Autodesk Inventor part; units mm, degrees
ref_plane "YZ Plane" through (0, 0, 0) normal (1, 0, 0) x (0, 1, 0)
ref_plane "XZ Plane" through (0, 0, 0) normal (0, 1, 0) x (-1, 0, 0)
ref_plane "XY Plane" through (0, 0, 0) normal (0, 0, 1) x (1, 0, 0)
sketch "Sketch1" plane through (0, 0, 0) normal (0, 0, 1) x (1, 0, 0)
  line L0 (0, 0) -> (479.525, 0)
  line L1 (479.525, 0) -> (479.525, 85)
  line L2 (479.525, 85) -> (0, 85)
  line L3 (0, 85) -> (0, 0)
  dimension "d0" = 479.525
  dimension "d1" = 85
extrude "Extrusion1" add sketch "Sketch1" along normal blind 4.7625
sketch "Sketch2" plane through (0, 0, 4.7625) normal (0, 0, 1) x (1, 0, 0)
  line L0 (0, 0) -> (479.525, 0)
  line L1 (382.925, 46.859) -> (382.925, 38.141)
  line L2 (399.525, 38.141) -> (399.525, 46.859)
  arc A0 (382.925, 38.141) -> (399.525, 38.141) centre (391.225, 42.5) ccw
  arc A1 (399.525, 46.859) -> (382.925, 46.859) centre (391.225, 42.5) ccw
  line L3 (479.525, 0) -> (479.525, 85)
  dimension "d5" = 16.6
  dimension "d6" = 9.375
  dimension "d7" = 9.375
  dimension "d8" = 42.5
  dimension "d23" = 80
extrude "Extrusion2" cut sketch "Sketch2" against normal up to next
sketch "Sketch3" plane through (0, 0, 4.7625) normal (0, 0, 1) x (1, 0, 0)
  line L0 (0, 0) -> (479.525, 0)
  line L1 (479.525, 0) -> (479.525, 85)
  line L2 (479.525, 85) -> (0, 85)
  line L3 (0, 85) -> (0, 0)
  circle A0 centre (14.7625, 75) radius 2.25
  circle A1 centre (14.7625, 10) radius 2.25
  circle A2 centre (464.7625, 75) radius 2.25
  circle A3 centre (464.7625, 10) radius 2.25
  circle A4 centre (238.2625, 10) radius 2.25
  circle A5 centre (238.2625, 75) radius 2.25
  dimension "d12" = 4.5
  dimension "d13" = 14.7625
  dimension "d14" = 14.7625
  dimension "d15" = 10
  dimension "d16" = 10
  dimension "d17" = 241.2625
extrude "Extrusion3" cut sketch "Sketch3" against normal up to next contours A0 | A1 | A2 | A3 | A4 | A5
chamfer "Chamfer1" distance 2 angle 45 6 edges at (236.0125, 75, 4.7625) (236.0125, 10, 4.7625) (462.5125, 10, 4.7625) (462.5125, 75, 4.7625) (12.5125, 75, 4.7625) (12.5125, 10, 4.7625)
properties part number "EnclosurePanelBottomFront" material "ABS Plastic"
Read the model definition and answer for the solid it produces. Units are mm, in the model's axes. Give positions to 0.01 mm unless a question says otherwise; leave off trailing zeros.
(1) Straight lines are drawn through the part: L1, parallel to Y at x = 236, z = 3.75; L2, parallel to Y at x = 398, z = 4.25. For each, find the intervals that lie inside material, in ascending order.
(2) Given pin 1 (12 mm diameter, centred on x = 367.5, y = 13, fed in from -Z); pin 2 (7 mm diameter, centred on x = 238.26, y = 10, fed in from +Z) (3 decimals); pin 3 (2.5 mm diameter, centred on x = 238.26, y = 75, fed in from -Z), each flat-ended and moving along its own axis, determine where each tip first touches the part or whether it passes through.
(3) For a pull along X with two mould halves and no side action, classify faces 1 (the flat face through (236, 43, 4.762)), 2 (the conical face through (15.9, 7.9, 2.9)) as released by +X, released by -X, zero draft, split by the parting line, or undercut.
Result sheet:
1. L1: y = 0 to 7.68, 12.32 to 72.68, 77.32 to 85
1. L2: y = 0 to 36.02, 48.98 to 85
2. pin 1: stops at z = 0
2. pin 2: stops at z = 4.015
2. pin 3: passes through
3. face 1: zero draft
3. face 2: undercut
